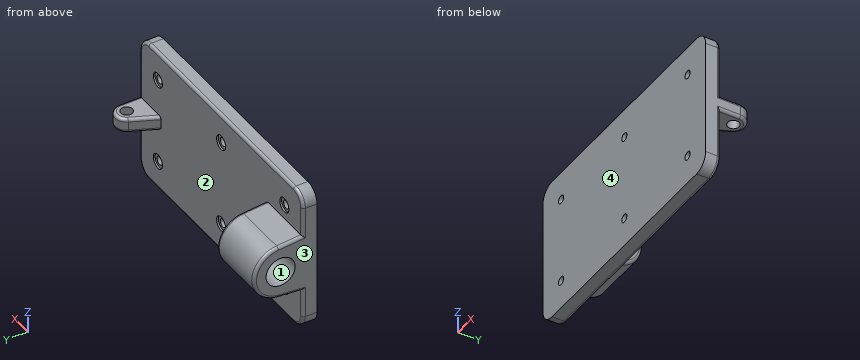
```python
from build123d import *

# Parameters (mm, degrees)
SKETCH1_W                      = 114.3
SKETCH1_H                      = 6.35
BASE_EXTRUDE_DEPTH             = 31.75
FILLET1_START                  = -3.175
FILLET1_DEPTH                  = 6.35
FILLET1_2_DEPTH                = 25.4
FILLET1_START_2                = -1
FILLET1_3_DEPTH                = 7.35
LEVER_BOSS_DEPTH               = 25.4
LEVER_BOSS_2_OUTLINE_W         = 6.35
LEVER_BOSS_2_OUTLINE_H         = 63.5
LEVER_BOSS_2_DEPTH             = 114.3
BOSS_EXTRUDE2_DEPTH            = 25.4
HOLE1_START                    = -1
HOLE1_DEPTH                    = 16.24
HOLE1_START_2                  = -3.175
HOLE1_2_OUTLINE_R              = 2.54
HOLE1_2_DEPTH                  = 6.35
HOLE2_D                        = 12.7
HOLE2_DEPTH                    = 25.4
F_4_SPOTFACE_HOLE1_D           = 3.6068
F_4_SPOTFACE_HOLE1_CBORE_D     = 6.35
F_4_SPOTFACE_HOLE1_CBORE_DEPTH = 0.762
LPATTERN1_COUNT                = 3
LPATTERN1_PITCH                = 44.45
LPATTERN1_COUNT_DIR2           = 2
LPATTERN1_PITCH_DIR2           = 38.1
FILLET2_R                      = 1.27


with BuildPart() as part:
    # Sketch1 → Base-Extrude (new, symmetric)
    with BuildSketch(Plane.XY):
        with Locations((57.15, 3.175)):
            Rectangle(SKETCH1_W, SKETCH1_H)
    extrude(amount=BASE_EXTRUDE_DEPTH, both=True)

    # Fillet1: read off the stored shape, not the designer's step
    # Fillet1 outline → Fillet1 (add)
    with BuildSketch(Plane.XY.offset(FILLET1_START)):
        with BuildLine():
            ThreePointArc((114.3, 15.24), (110.319513239, 20.199583716), (104.615956442, 17.38690077))
            Line((104.615956442, 17.38690077), (99.469365091, 6.35))
            Line((99.469365091, 6.35), (114.3, 6.35))
            Line((114.3, 6.35), (114.3, 15.24))
        make_face()
    extrude(amount=FILLET1_DEPTH)

    # Fillet1 2 outline → Fillet1 2 (add)
    with BuildSketch(Plane.YZ):
        with BuildLine():
            Line((6.35, -12.7), (16.905312852, -11.776529785))
            ThreePointArc((16.905312852, -11.776529785), (27.696514216, 0), (16.905312852, 11.776529785))
            Line((16.905312852, 11.776529785), (6.35, 12.7))
            Line((6.35, 12.7), (6.35, -12.7))
        make_face()
    extrude(amount=FILLET1_2_DEPTH)

    # Fillet1 3 outline → Fillet1 3 (cut)
    with BuildSketch(Plane(origin=(0, 0, 0), x_dir=(1, 0, 0), z_dir=(0, 1, 0)).offset(FILLET1_START_2)):
        with BuildLine():
            ThreePointArc((0, 25.4), (1.859871939, 29.890128061), (6.35, 31.75))
            Line((6.35, 31.75), (0, 31.75))
            Line((0, 31.75), (0, 25.4))
        make_face()
        with BuildLine():
            Line((114.3, 31.75), (107.95, 31.75))
            ThreePointArc((107.95, 31.75), (112.440128061, 29.890128061), (114.3, 25.4))
            Line((114.3, 25.4), (114.3, 31.75))
        make_face()
        with BuildLine():
            ThreePointArc((6.35, -31.75), (1.859871939, -29.890128061), (0, -25.4))
            Line((0, -25.4), (0, -31.75))
            Line((0, -31.75), (6.35, -31.75))
        make_face()
        with BuildLine():
            ThreePointArc((114.3, -25.4), (112.440128061, -29.890128061), (107.95, -31.75))
            Line((107.95, -31.75), (114.3, -31.75))
            Line((114.3, -31.75), (114.3, -25.4))
        make_face()
    extrude(amount=FILLET1_3_DEPTH, mode=Mode.SUBTRACT)

    # lever boss: read off the stored shape, not the designer's step
    # lever boss outline → lever boss (cut)
    with BuildSketch(Plane.YZ):
        with BuildLine():
            Line((16.905312852, 11.776529785), (6.35, 12.7))
            Line((6.35, 12.7), (6.35, -12.7))
            Line((6.35, -12.7), (16.905312852, -11.776529785))
            ThreePointArc((16.905312852, -11.776529785), (27.696514216, 0), (16.905312852, 11.776529785))
        make_face()
    extrude(amount=LEVER_BOSS_DEPTH, mode=Mode.SUBTRACT)

    # lever boss 2 outline → lever boss 2 (add)
    with BuildSketch(Plane.YZ):
        with Locations((3.175, 0)):
            Rectangle(LEVER_BOSS_2_OUTLINE_W, LEVER_BOSS_2_OUTLINE_H)
    extrude(amount=LEVER_BOSS_2_DEPTH)

    # Sketch3 → Boss-Extrude2 (add)
    with BuildSketch(Plane.ZY):
        with BuildLine():
            Line((12.7, 6.35), (11.776529785, 16.905312852))
            ThreePointArc((11.776529785, 16.905312852), (0, 27.696514216), (-11.776529785, 16.905312852))
            Line((-11.776529785, 16.905312852), (-12.7, 6.35))
            Line((-12.7, 6.35), (12.7, 6.35))
        make_face()
    extrude(amount=-BOSS_EXTRUDE2_DEPTH)

    # Hole1: read off the stored shape, not the designer's step
    # Hole1 outline → Hole1 (cut)
    with BuildSketch(Plane(origin=(0, 0, 0), x_dir=(1, 0, 0), z_dir=(0, 1, 0)).offset(HOLE1_START)):
        with BuildLine():
            ThreePointArc((0, 25.4), (1.859871939, 29.890128061), (6.35, 31.75))
            Line((6.35, 31.75), (0, 31.75))
            Line((0, 31.75), (0, 25.4))
        make_face()
        with BuildLine():
            Line((114.3, 31.75), (107.95, 31.75))
            ThreePointArc((107.95, 31.75), (112.440128061, 29.890128061), (114.3, 25.4))
            Line((114.3, 25.4), (114.3, 31.75))
        make_face()
        with BuildLine():
            ThreePointArc((6.35, -31.75), (1.859871939, -29.890128061), (0, -25.4))
            Line((0, -25.4), (0, -31.75))
            Line((0, -31.75), (6.35, -31.75))
        make_face()
        with BuildLine():
            ThreePointArc((114.3, -25.4), (112.440128061, -29.890128061), (107.95, -31.75))
            Line((107.95, -31.75), (114.3, -31.75))
            Line((114.3, -31.75), (114.3, -25.4))
        make_face()
    extrude(amount=HOLE1_DEPTH, mode=Mode.SUBTRACT)

    # Hole1 2 outline → Hole1 2 (cut)
    with BuildSketch(Plane.XY.offset(HOLE1_START_2)):
        with Locations((109.22, 15.24)):
            Circle(HOLE1_2_OUTLINE_R)
    extrude(amount=HOLE1_2_DEPTH, mode=Mode.SUBTRACT)

    # Hole2
    with Locations(Plane(origin=(25.4, 3.190032044, 95.175064019), x_dir=(0, 0, -1), z_dir=(1, 0, 0))):
        with Locations((95.175064019, 12.684967956)):
            Hole(HOLE2_D / 2, depth=HOLE2_DEPTH)

    # #4 spotface hole1 (through all)
    with Locations(Plane(origin=(72.288522493, 6.35, 6.630777087), x_dir=(-1, 0, 0), z_dir=(0, 1, 0))):
        with Locations((-29.311477507, 12.419222913)):
            f_4_spotface_hole1 = CounterBoreHole(F_4_SPOTFACE_HOLE1_D / 2, F_4_SPOTFACE_HOLE1_CBORE_D / 2, F_4_SPOTFACE_HOLE1_CBORE_DEPTH)

    # LPattern1: 4 spotface hole1 3 × 2
    with Locations(*[(-i * LPATTERN1_PITCH, 0, -j * LPATTERN1_PITCH_DIR2) for i in range(LPATTERN1_COUNT) for j in range(LPATTERN1_COUNT_DIR2) if (i, j) != (0, 0)]):
        add(f_4_spotface_hole1, mode=Mode.SUBTRACT)

    # Fillet2
    fillet2_edges = [part.edges().sort_by_distance(p)[0] for p in [
        (114.3, 6.35, -14.2875),
        (114.3, 10.795, -3.175),
        (110.319513239, 20.199583716, -3.175),
        (102.042660767, 11.868450385, -3.175),
        (114.3, 10.795, 3.175),
        (110.319513239, 20.199583716, 3.175),
        (102.042660767, 11.868450385, 3.175),
        (0, 6.35, -19.05),
        (0, 11.627656426, -12.238264893),
        (0, 27.696514216, 0),
        (25.4, 11.627656426, 12.238264893),
        (25.4, 11.627656426, -12.238264893),
        (25.4, 27.696514216, 0),
        (0, 11.627656426, 12.238264893),
        (57.15, 6.35, -31.75),
        (57.15, 6.35, 31.75),
        (112.440128061, 6.35, -29.890128061),
        (112.440128061, 6.35, 29.890128061),
        (1.859871939, 6.35, 29.890128061),
        (1.859871939, 6.35, -29.890128061),
    ]]
    fillet(fillet2_edges, radius=FILLET2_R)


solid = part.part
```
Verification items for the finished model (mm, model axes). Face numbers are marked on the shaded views. Give positions to 0.01 mm unless a question says otherwise; leave off trailing zeros. Loops run counter-clockwise (first coordinate to the right, second up) from the corner with the lowest first, then second, coordinate; pieces in that order, holes last. Notation, with made-up numbers: M 62.5,69 L 83.5,69 A12 ccw 83.5,77 Z; hole C 3,75 d8. An arc over 180 degrees is marked long. Return JSON: item names as keys, results as strings.
1) Gauge pin test, flat ends, axial feed: P1, Ø4.5, axis at x = 12.7, z = 19.05, coming from the -Y side; P2, Ø3, axis at x = 67.5, z = -13, coming from the +Y side; P3, Ø3.5, axis at x = 105, y = 13, coming from the -Z side (3 decimals); P4, Ø1.9, axis at x = 56, z = -20, coming from the +Y side. Record the tip position at first contact, or that the pin passes through.
Findings:
{"P1": "stops at y = 0", "P2": "stops at y = 6.35", "P3": "stops at z = -3.175", "P4": "stops at y = 5.59"}
2) Section check B-B, the plane x = 12.7. Enter the section's corners in (y, z) (3 decimals).
Findings:
{"outline": "M 0,-31.75 L 5.08,-31.75 A1.27 ccw 6.35,-30.48 L 6.35,-22.225 L 5.588,-22.225 L 5.588,-20.853 L 0,-20.853 Z; M 0,-17.247 L 5.588,-17.247 L 5.588,-15.875 L 6.35,-15.875 L 6.35,-12.7 L 16.905,-11.777 A11.822 ccw 16.905,11.777 L 6.35,12.7 L 6.35,15.875 L 5.588,15.875 L 5.588,17.247 L 0,17.247 Z; M 0,20.853 L 5.588,20.853 L 5.588,22.225 L 6.35,22.225 L 6.35,30.48 A1.27 ccw 5.08,31.75 L 0,31.75 Z; hole C 15.875,0 d12.7"}
3) Section check C-C, the plane x = 57.15. Enter the section's corners in (y, z) (3 decimals).
Findings:
{"outline": "M 0,-31.75 L 5.08,-31.75 A1.27 ccw 6.35,-30.48 L 6.35,-22.225 L 5.588,-22.225 L 5.588,-20.853 L 0,-20.853 Z; M 0,-17.247 L 5.588,-17.247 L 5.588,-15.875 L 6.35,-15.875 L 6.35,15.875 L 5.588,15.875 L 5.588,17.247 L 0,17.247 Z; M 0,20.853 L 5.588,20.853 L 5.588,22.225 L 6.35,22.225 L 6.35,30.48 A1.27 ccw 5.08,31.75 L 0,31.75 Z"}
4) Material ranges on L1, parallel to Z at x = 57.15, y = 1.95; L2, parallel to Y at x = 74.5, z = 12.5, recorded low to high. Write a range as [from, to].
Findings:
{"L1": "z = [-31.75, -20.85], [-17.25, 17.25], [20.85, 31.75]", "L2": "y = [0, 6.35]"}
5) Mould release check, pull along Y, two halves, no side actions. Record for the marked faces 1, 2, 3 and 4: released by +Y, released by -Y, zero draft, split by the parting line, or undercut.
Findings:
{"face 1": "undercut", "face 2": "released by +Y", "face 3": "zero draft", "face 4": "released by -Y"}
6) Section check A-A, the plane z = 0. Enter the section's corners in (x, y) (3 decimals), and give its area (3 significant figures).
Findings:
{"outline": "M 0,0 L 114.3,0 L 114.3,15.24 A5.08 ccw 104.616,17.387 L 99.469,6.35 L 25.4,6.35 L 25.4,9.525 L 0,9.525 Z; M 0,22.225 L 25.4,22.225 L 25.4,26.427 A1.27 ccw 24.13,27.697 L 1.27,27.697 A1.27 ccw 0,26.427 Z; hole C 109.22,15.24 d5.08", "area": "1,080 mm2"}
7) Section check D-D, the plane z = 19.05. Count the separate pieces of the cut face and the enclosed holes in it, and give its area (3 significant figures).
Findings:
{"separate pieces": "4", "enclosed holes": "0", "area": "650 mm2"}
